Read the model definition and answer for the solid it produces. Units are mm, in the model's axes. A direction names the side the tool comes from. Coordinates: 2 decimals unless noted, no trailing zeros. Write each loop counter-clockwise with the first axis right and the second up, starting at its lowest first coordinate (ties: lowest second). Pieces come first, ordered by that corner, then holes. Notation, with made-up numbers: (-32.75, 27) -> (-21.75, 27) arc R21 cw to (-21.75, 52) -> close; hole circle Ø6 at (59.5, 56). An arc over 180 degrees is marked (long way). One line per item, written item: value. Start each with the question number.
from build123d import *

# Parameters (mm, degrees)
F1_DEPTH = 63.5
F2_DEPTH = 25.4
F3_DEPTH = 12.7
F0_W     = 25.4
F0_H     = 19.05
F4_DEPTH = 25.4
F6_R     = 6.35


with BuildPart() as f1:
    # F0 (on Front) → F1 (new body, symmetric)
    with BuildSketch(Plane.XZ):
        Polygon((41.275, -9.525), (41.275, 9.525), (22.225, 9.525), (-41.275, 9.525), (-41.275, -9.525), align=None)
    extrude(amount=F1_DEPTH, both=True)

    # F0 (on Front) → F2 (join, symmetric)
    with BuildSketch(Plane.XZ):
        with BuildLine():
            Line((22.225, 9.525), (41.275, 9.525))
            Line((41.275, 9.525), (41.275, 27.0002))
            ThreePointArc((41.275, 27.0002), (45.9246798487, 38.2255201513), (57.15, 42.8752))
            Line((57.15, 42.8752), (60.325, 42.8752))
            Line((60.325, 42.8752), (60.325, 61.9252))
            Line((60.325, 61.9252), (57.15, 61.9252))
            add(Edge.make_bspline(
                [(56.0630860739, 61.9082827763), (56.4239855427, 61.9164147912), (56.7862841158, 61.9220646594), (57.15, 61.9252)],
                knots=[110.5496251445, 110.5496251445, 110.5496251445, 110.5496251445, 111.5045361635, 111.5045361635, 111.5045361635, 111.5045361635], degree=3))
            ThreePointArc((56.0630860739, 61.9082827763), (32.0729577714, 51.3085849333), (22.225, 27.0002))
            Line((22.225, 27.0002), (22.225, 9.525))
        make_face()
    extrude(amount=F2_DEPTH, both=True)

    # F0 (on Front) → F3 (join, symmetric)
    with BuildSketch(Plane.XZ):
        with BuildLine():
            Line((-41.275, 9.525), (22.225, 9.525))
            Line((22.225, 9.525), (22.225, 27.0002))
            ThreePointArc((22.225, 27.0002), (32.0729577714, 51.3085849333), (56.0630860739, 61.9082827763))
            add(Edge.make_bspline(
                [(-41.275, 9.525), (-8.7476331645, 26.7582086028), (14.2819146452, 60.9668430208), (56.0630860739, 61.9082827763)],
                knots=[0, 0, 0, 0, 110.5496251445, 110.5496251445, 110.5496251445, 110.5496251445], degree=3))
        make_face()
    extrude(amount=F3_DEPTH, both=True)

    # F0 (on Front) → F4 (join, symmetric)
    with BuildSketch(Plane.XZ):
        with Locations((73.025, 52.4002)):
            Rectangle(F0_W, F0_H)
    extrude(amount=F4_DEPTH, both=True)

    # F0 (on Front) → F5 (revolve)
    with BuildSketch(Plane.XZ):
        Polygon((85.725, 61.9252), (85.725, 42.8752), (85.725, 38.1), (111.125, 38.1), (111.125, 66.675), (85.725, 66.675), align=None)
    revolve(axis=Axis((85.725, 0, 52.3875), (0, 0, -1)))

    # F6
    f6_edges = [f1.edges().sort_by_distance(p)[0] for p in [
        (41.275, -63.5, 0),
        (-41.275, -63.5, 0),
        (-41.275, 63.5, 0),
        (41.275, 63.5, 0),
    ]]
    fillet(f6_edges, radius=F6_R)


solid = f1.part
1. A cutting plane is placed at A-A on z = -1.5. Give the vertices of the cut face in (x, y) (3 decimals).
2. Given pin 1 (15.5 mm diameter, centred on x = 68, z = 38.5, fed in from +Y); pin 2 (23 mm diameter, centred on x = 76, y = 10, fed in from -Z); pin 3 (6 mm diameter, centred on x = 57, y = 8, fed in from +Z), each flat-ended and moving along its own axis, determine where each tip first touches the part or whether it passes through.
3. For a pull along X with two mould halves and no side action, classify faces 1 (the face through (39.464, -61.59, 0.133)), 2 (the face through (60, 2, 61.925)), 3 (the face through (45.8, -0.4, 38.1)), 4 (the face through (-39.464, -61.59, -0.133)) as +X half, -X half, draft (parallel to the pull), parting line (faces both ways), or undercut.
4. A tool of negligible diameter and unlimited length cuts with its end or side. For faces 5 (the face through (86, 0, 38.1)), 6 (the face through (32.34, 18.96, 51.58)), 7 (the face through (46, 25.4, 42)), 8 (the face through (1, -38, 9.525)), from which of +Z, -Z, +X, -X, +Y, -Y can it reach the whole face along a straight path? Write none if from no direction.
5. A cutting plane is placed at B-B on x = 79. Give the vertices of the cut face in (y, z) (3 decimals).
6. Find the intervals of material crossed by probe 1 along Z at (x, y) = (14, 43.5) (3 decimals); probe 2 along X at (y, z) = (-25, -4.5) (3 decimals); probe 3 along Y at (x, z) = (24.5, 53), in increasing order. Write a range as from..to.
Derived:
1. outline: (-41.275, -57.15) arc R6.35 ccw to (-34.925, -63.5) -> (34.925, -63.5) arc R6.35 ccw to (41.275, -57.15) -> (41.275, 57.15) arc R6.35 ccw to (34.925, 63.5) -> (-34.925, 63.5) arc R6.35 ccw to (-41.275, 57.15) -> close
2. pin 1: stops at y = 25.4
2. pin 2: stops at z = 38.1
2. pin 3: stops at z = 61.93
3. face 1: +X half
3. face 2: draft
3. face 3: undercut
3. face 4: -X half
4. face 5: -Z, +X, +Y, -Y
4. face 6: +Z, -X, +Y
4. face 7: +Z, +X, -X, +Y
4. face 8: +Z, -X, -Y
5. outline: (-25.4, 42.875) -> (-24.494, 42.875) -> (-24.494, 38.1) -> (24.494, 38.1) -> (24.494, 42.875) -> (25.4, 42.875) -> (25.4, 61.925) -> (24.494, 61.925) -> (24.494, 66.675) -> (-24.494, 66.675) -> (-24.494, 61.925) -> (-25.4, 61.925) -> close
6. probe 1: z = -9.525..9.525
6. probe 2: x = -41.275..41.275
6. probe 3: y = -12.7..12.7
